from build123d import *

# Parameters (mm, degrees)
SKETCH1_R           = 3.25
BOSS_EXTRUDE1_DEPTH = 22.686
SKETCH6_R           = 4.7
BOSS_EXTRUDE2_DEPTH = 8
FILLET2_R           = 0.75
SKETCH7_R           = 1.5
BOSS_EXTRUDE3_DEPTH = 1
BOSS_EXTRUDE4_DEPTH = 2


with BuildPart() as part:
    # Sketch1 → Boss-Extrude1 (new body)
    with BuildSketch(Plane(origin=(0, 0, 0), x_dir=(1, 0, 0), z_dir=(0, 1, 0))):
        Circle(SKETCH1_R)
    extrude(amount=BOSS_EXTRUDE1_DEPTH)

    # Sketch6 → Boss-Extrude2 (add)
    with BuildSketch(Plane(origin=(0, 22.686, 0), x_dir=(1, 0, 0), z_dir=(0, 1, 0))):
        Circle(SKETCH6_R)
    extrude(amount=BOSS_EXTRUDE2_DEPTH)

    # Fillet2
    fillet2_edges = [part.edges().sort_by_distance(p)[0] for p in [
        (-4.7, 30.686, 0),
    ]]
    fillet(fillet2_edges, radius=FILLET2_R)

    # Sketch7 → Boss-Extrude3 (add)
    with BuildSketch(Plane(origin=(0, 30.686, 0), x_dir=(1, 0, 0), z_dir=(0, 1, 0))):
        Circle(SKETCH7_R)
    extrude(amount=BOSS_EXTRUDE3_DEPTH)

    # Sketch8 → Boss-Extrude4 (add)
    with BuildSketch(Plane.XZ.offset(-22.686)):
        with BuildLine():
            Line((-1.016, 4.588871757), (-1.016, 6.620871757))
            Line((-1.016, 6.620871757), (1.016, 6.620871757))
            Line((1.016, 6.620871757), (1.016, 4.588871757))
            ThreePointArc((1.016, 4.588871757), (0, 4.7), (-1.016, 4.588871757))
        make_face()
        with BuildLine():
            Line((1.016, -6.620871757), (1.016, -4.588871757))
            ThreePointArc((1.016, -4.588871757), (0, -4.7), (-1.016, -4.588871757))
            Line((-1.016, -4.588871757), (-1.016, -6.620871757))
            Line((-1.016, -6.620871757), (1.016, -6.620871757))
        make_face()
    extrude(amount=-BOSS_EXTRUDE4_DEPTH)


solid = part.part
Read the model definition and answer for the solid it produces. Units are mm, in the model's axes. A direction names the side the tool comes from. Coordinates: 2 decimals unless noted, no trailing zeros. Loops run counter-clockwise (first coordinate to the right, second up) from the corner with the lowest first, then second, coordinate; pieces in that order, holes last. Notation, with made-up numbers: (-32, 51) -> (14, 51) arc R16 cw to (14, 79) -> close; hole circle Ø1 at (14, 38). An arc over 180 degrees is marked (long way). Write item = value, one per line. Start each with the question number.
1) The part is cut by section D-D, the plane z = 5.25. Determine the outline of the cut face in (x, y).
2) The part is cut by section B-B, the plane x = 0. Determine the outline of the cut face in (y, z).
3) The part is cut by section C-C, the plane y = 24. Determine the outline of the cut face in (x, z), plus the area to 3 significant figures.
4) For faces 1 (the face through (-1.016, 24, 6)), 2 (the face through (-1.016, 24, -6)), 3 (the face through (-1.5, 31.18, -0.07)), 4 (the face through (1.016, 24, 6)), 5 (the face through (1.016, 24, -6)), determine the directions among +Z, -Z, +X, -X, +Y, -Y from which every point of the face is accessible in a straight line to the end or side of a thin tool.
5) The part is cut by section A-A, the plane z = 0. Determine the outline of the cut face in (x, y), plus the area to 3 significant figures.
6) Given P1, Ø1.6, axis at y = 23.5, z = -5.5, coming from the -X side; P2, Ø1, axis at x = -0.5, z = -5.5, coming from the +Y side; P3, Ø0.6, axis at y = 23, z = -5.5, coming from the +X side; P4, Ø4, axis at x = 2.5, z = -1, coming from the +Y side, each flat-ended and moving along its own axis, determine where each tip first touches the part or whether it passes through.
7) Find the intervals of material crossed by L1, parallel to Y at x = -1, z = -2.5; L2, parallel to Y at x = -0.75, z = -5.5; L3, parallel to Z at x = 0.75, y = 7, in increasing order. Write a range as from..to.
Result:
q1.outline = (-1.02, 22.69) -> (1.02, 22.69) -> (1.02, 24.69) -> (-1.02, 24.69) -> close
q2.outline = (0, -3.25) -> (22.69, -3.25) -> (22.69, -6.62) -> (24.69, -6.62) -> (24.69, -4.7) -> (29.94, -4.7) arc R0.75 ccw to (30.69, -3.95) -> (30.69, -1.5) -> (31.69, -1.5) -> (31.69, 1.5) -> (30.69, 1.5) -> (30.69, 3.95) arc R0.75 ccw to (29.94, 4.7) -> (24.69, 4.7) -> (24.69, 6.62) -> (22.69, 6.62) -> (22.69, 3.25) -> (0, 3.25) -> close
q3.outline = (-1.02, -6.62) -> (1.02, -6.62) -> (1.02, -4.59) arc R4.7 ccw to (1.02, 4.59) -> (1.02, 6.62) -> (-1.02, 6.62) -> (-1.02, 4.59) arc R4.7 ccw to (-1.02, -4.59) -> close
q3.area = 77.4 mm²
q4.face_1 = +Z, -X, +Y, -Y
q4.face_2 = -Z, -X, +Y, -Y
q4.face_3 = +Y
q4.face_4 = +Z, +X, +Y, -Y
q4.face_5 = -Z, +X, +Y, -Y
q5.outline = (-4.7, 22.69) -> (-3.25, 22.69) -> (-3.25, 0) -> (3.25, 0) -> (3.25, 22.69) -> (4.7, 22.69) -> (4.7, 29.94) arc R0.75 ccw to (3.95, 30.69) -> (1.5, 30.69) -> (1.5, 31.69) -> (-1.5, 31.69) -> (-1.5, 30.69) -> (-3.95, 30.69) arc R0.75 ccw to (-4.7, 29.94) -> close
q5.area = 225 mm²
q6.P1 = -1.02
q6.P2 = 24.69
q6.P3 = 1.02
q6.P4 = 31.69
q7.L1 = 0..30.69
q7.L2 = 22.69..24.69
q7.L3 = -3.16..3.16
